Autodesk Inventor part; units mm, degrees
ref_plane "YZ Plane" through (0, 0, 0) normal (1, 0, 0) x (0, 1, 0)
ref_plane "XZ Plane" through (0, 0, 0) normal (0, 1, 0) x (-1, 0, 0)
ref_plane "XY Plane" through (0, 0, 0) normal (0, 0, 1) x (1, 0, 0)
sketch "Boceto1" plane through (0, 0, 0) normal (1, 0, 0) x (0, 1, 0)
  circle A0 centre (0, 0) radius 9.5
  circle A1 centre (0, 0) radius 5.5
  dimension "d0" = 19
  dimension "d1" = 11
extrude "Extrusión1" add sketch "Boceto1" along normal mid plane 70 contours A1
extrude "Extrusión2" add sketch "Boceto1" along normal mid plane 30
properties part number "Bracket polea"
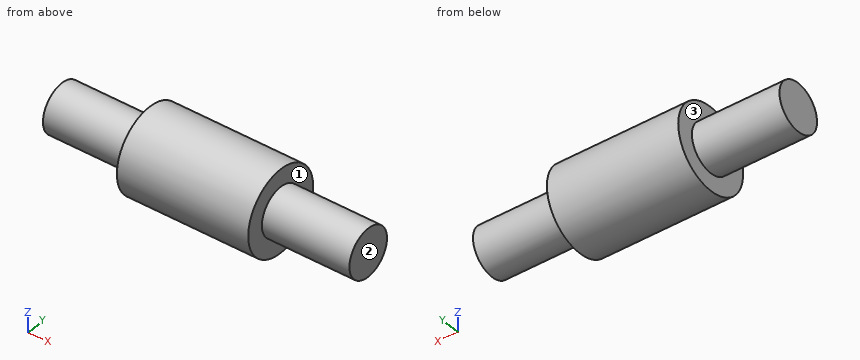
Work out the finished part from the listing and answer in its coordinate system (mm). Face numbers are marked on the shaded views. A direction names the side the tool comes from. Round coordinates to 2 decimals unless told otherwise and drop trailing zeros. Write each loop counter-clockwise with the first axis right and the second up, starting at its lowest first coordinate (ties: lowest second). Pieces come first, ordered by that corner, then holes.
1) Consider probe 1 along X at (y, z) = (2.75, -7.5); probe 2 along Z at (x, y) = (-5.5, 7.75); probe 3 along Z at (x, y) = (-2, 6.25). Determine where each line is inside the solid, lowest interval first.
2) A cutting plane is placed at D-D on x = -22. Determine the outline of the cut face in (y, z), and give its area (3 significant figures).
3) A cutting plane is placed at A-A on y = 0. Determine the outline of the cut face in (x, z), and give its area (3 significant figures).
4) Which of the six approach directions +Z, -Z, +X, -X, +Y, -Y give full straight-line access (tool end or side, diameter ignored) to the marked faces 1, 2 and 3?
5) A cutting plane is placed at C-C on x = 11. Determine the outline of the cut face in (y, z).
6) Flat-ended cylindrical pins translate along their axes: P1, Ø1, axis at x = -23, z = -4, coming from the +Y side; P2, Ø1, axis at x = -14.5, y = -2, coming from the -Z side; P3, Ø5, axis at x = -7.5, z = -4, coming from the +Y side. Find the tip coordinate at first contact, or state that the pin passes through.
Entries:
1. probe 1: x = -15 to 15
1. probe 2: z = -5.49 to 5.49
1. probe 3: z = -7.15 to 7.15
2. outline: circle Ø11 at (0, 0)
2. area: 95.0 mm2
3. outline: (-35, -5.5) - (-15, -5.5) - (-15, -9.5) - (15, -9.5) - (15, -5.5) - (35, -5.5) - (35, 5.5) - (15, 5.5) - (15, 9.5) - (-15, 9.5) - (-15, 5.5) - (-35, 5.5) - close
3. area: 1,010 mm2
4. face 1: +X
4. face 2: +Z, -Z, +X, +Y, -Y
4. face 3: -X
5. outline: circle Ø19 at (0, 0)
6. P1: stops at y = 4.24
6. P2: stops at z = -9.38
6. P3: stops at y = 9.38
